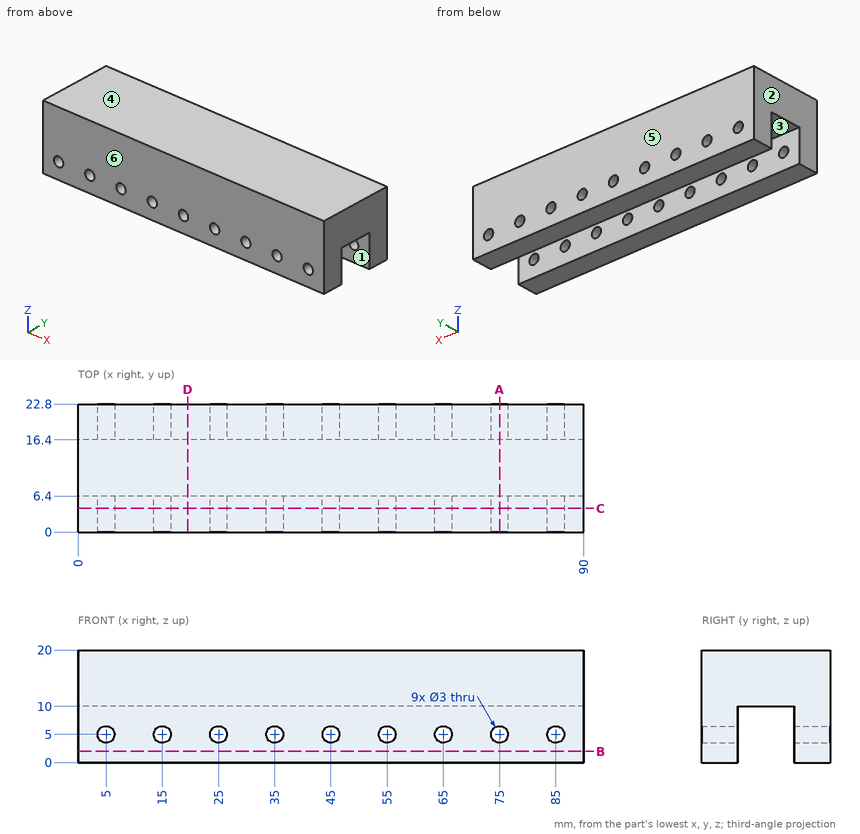
Here's the drawing with two shaded views (mm, measured from the low corner). I have some questions. A direction names the side the tool comes from. Coordinates: 2 decimals unless noted, no trailing zeros. Order: outer loops, then holes, each group sorted by start corner. A loop starts at its lowest first (then second) coordinate and runs counter-clockwise, first axis right, second up. Notation, with made-up numbers: (61, 75) -> (107, 75) arc R17 cw to (107, 104) -> close; hole circle Ø10 at (59, 64.25). An arc over 180 degrees is marked (long way). One line per question, with ' | ' between items.
Q1. On a 3-axis mill with a long thin cutter (end or side, diameter ignored), from which of +Z, -Z, +X, -X, +Y, -Y can I reach the whole of each face in a straight line? I mean the marked faces 1 and 2. Say none if no direction works.
Return value:
face 1: -Z, +X, -X | face 2: +Z, -Z, -X, +Y, -Y
Q2. Thinking about a two-plate mould opening in Y: for the marked faces 3, 4, 5 and 6, which applies, pulls with the +Y half, pulls with the -Y half, needs draft (parallel to the pull), parting line crosses it, or undercut?
Return value:
face 3: undercut | face 4: needs draft | face 5: pulls with the +Y half | face 6: pulls with the -Y half
Q3. Imagine slicing it at C-C on y = 4.25. State how many separate pieces and enclosed holes the cut face has, and give its area (3 significant figures).
Return value:
separate pieces: 1 | enclosed holes: 9 | area: 1,740 mm²
Q4. Imagine slicing it at A-A on x = 75. Please give me the cut outline in (y, z), and give its area (3 significant figures).
Return value:
outline: (0, 0) -> (6.4, 0) -> (6.4, 3.5) -> (0, 3.5) -> close; (0, 6.5) -> (6.4, 6.5) -> (6.4, 10) -> (16.4, 10) -> (16.4, 6.5) -> (22.8, 6.5) -> (22.8, 20) -> (0, 20) -> close; (16.4, 0) -> (22.8, 0) -> (22.8, 3.5) -> (16.4, 3.5) -> close | area: 318 mm²
Q5. Imagine slicing it at B-B on z = 2. Please give me the cut outline in (x, y), and give its area (3 significant figures).
Return value:
outline: (0, 0) -> (90, 0) -> (90, 6.4) -> (0, 6.4) -> close; (0, 16.4) -> (90, 16.4) -> (90, 22.8) -> (0, 22.8) -> close | area: 1,150 mm²
Q6. If I drill on L1, parallel to Y at x = 4, z = 6.75; L2, parallel to Z at x = 65, y = 2; L3, parallel to Z at x = 24.5, y = 6.5, over which ranges is the centre line in solid material (lowest first)?
Return value:
L1: 0 to 6.4, 16.4 to 22.8 | L2: 0 to 3.5, 6.5 to 20 | L3: 10 to 20
Q7. Imagine slicing it at D-D on x = 19.5. Please give me the cut outline in (y, z), and give its area (3 significant figures).
Return value:
outline: (0, 0) -> (6.4, 0) -> (6.4, 10) -> (16.4, 10) -> (16.4, 0) -> (22.8, 0) -> (22.8, 20) -> (0, 20) -> close | area: 356 mm²
Q8. I'm going to push a flat-ended pin straight in: P1, Ø1, axis at x = 62, y = 11, coming from the -Z side. Where does the tip first touch, or does it pass through?
Return value:
P1: z = 10
